```python
from build123d import *

# Parameters (mm, degrees)
SKETCH1_W           = 70
SKETCH1_H           = 60
BOSS_EXTRUDE1_DEPTH = 5.7
SKETCH2_W           = 10
SKETCH2_H           = 60
SKETCH2_R           = 2.25
BOSS_EXTRUDE2_DEPTH = 3.3
FILLET1_R           = 5
SKETCH2_4_R         = 2.5
CUT_EXTRUDE2_DEPTH  = 5


with BuildPart() as part:
    # Sketch1 → Boss-Extrude1 (new body)
    with BuildSketch(Plane(origin=(0, 0, 0), x_dir=(1, 0, 0), z_dir=(0, 1, 0))):
        Rectangle(SKETCH1_W, SKETCH1_H)
    extrude(amount=BOSS_EXTRUDE1_DEPTH)

    # Sketch2 → Boss-Extrude2 (add)
    # profile 1 of 2: a face of its own
    with BuildSketch(Plane(origin=(0, 5.7, 0), x_dir=(1, 0, 0), z_dir=(0, 1, 0))):
        with Locations((-30, 0)):
            Rectangle(SKETCH2_W, SKETCH2_H)
        with Locations(Location((-30, -25, 0), (0, 0, 270))):
            Circle(SKETCH2_R, mode=Mode.SUBTRACT)
        with Locations(Location((-30, 25, 0), (0, 0, 270))):
            Circle(SKETCH2_R, mode=Mode.SUBTRACT)
    # profile 2 of 2: a face of its own
    with BuildSketch(Plane(origin=(0, 5.7, 0), x_dir=(1, 0, 0), z_dir=(0, 1, 0))):
        with Locations((30, 0)):
            Rectangle(SKETCH2_W, SKETCH2_H)
        with Locations(Location((30, -25, 0), (0, 0, 270))):
            Circle(SKETCH2_R, mode=Mode.SUBTRACT)
        with Locations(Location((30, 25, 0), (0, 0, 90))):
            Circle(SKETCH2_R, mode=Mode.SUBTRACT)
    extrude(amount=BOSS_EXTRUDE2_DEPTH)

    # Fillet1
    fillet1_edges = [part.edges().sort_by_distance(p)[0] for p in [
        (-35, 4.5, -30),
        (-35, 4.5, 30),
        (35, 4.5, 30),
        (35, 4.5, -30),
    ]]
    fillet(fillet1_edges, radius=FILLET1_R)

    # Sketch2_4 → Cut-Extrude2 (cut)
    with BuildSketch(Plane(origin=(0, 5.7, 0), x_dir=(1, 0, 0), z_dir=(0, 1, 0))):
        with Locations(Location((-9, 5, 0), (0, 0, 270))):
            Circle(SKETCH2_4_R)
        with Locations(Location((9, 5, 0), (0, 0, 270))):
            Circle(SKETCH2_4_R)
    extrude(amount=-CUT_EXTRUDE2_DEPTH, mode=Mode.SUBTRACT)


solid = part.part
```
CAD build for the part. Positions are in the model's coordinates, mm. A direction names the side the tool comes from. Round coordinates to 2 decimals unless told otherwise and drop trailing zeros. Order: outer loops, then holes, each group sorted by start corner. A loop starts at its lowest first (then second) coordinate and runs counter-clockwise, first axis right, second up. Notation, with made-up numbers: (46.5, 8) - (62.5, 8) arc R19 cw to (62.5, 15) - close; hole circle Ø4 at (27, 15). An arc over 180 degrees is marked (long way). Answer in a Markdown table with one row per item. Add a question column.
(1) Probe L1, parallel to X at y = 1.85, z = -5; L2, parallel to X at y = 7.75, z = -1; L3, parallel to X at y = 6, z = 24.5. List the from-to ranges inside material, lowest first. Write a range as [from, to].
(2) Drop flat-ended pins along their axis: pin 1 Ø4 at (x, z) = (-8, -5) entering from +Y; pin 2 Ø7 at (x, z) = (-30, -25) entering from -Y; pin 3 Ø4 at (x, z) = (-9, -5) entering from +Y. Give the stop position or say it passes through.
(3) Mould opens along Z. For faces 1 (the face through (30, 5.7, 25)), 2 (the face through (-34, 5, 28)), 3 (the face through (-30, 9, 0)) say: +Z half, -Z half, draft (parallel to the pull), parting line (faces both ways), or undercut.
(4) 3-axis set-ups, long thin cutter, end or side, ignore diameter. For faces 4 (the face through (-31.996, 7.327, -23.962)), 5 (the face through (-35, 4, 0)), 6 (the face through (0, 5.7, 0)): which of +Z, -Z, +X, -X, +Y, -Y reach the whole face in a straight line?
(5) Band-saw the part on C-C on z = 20. List the corners of the cut face in (x, y).
(6) Band-saw the part on B-B on x = -9. List the corners of the cut face in (y, z), and give its area (3 significant figures).
(7) Band-saw the part on A-A on y = 6.5. List the corners of the cut face in (x, z).
(8) Band-saw the part on D-D on z = -5. List the corners of the cut face in (x, y).
Data:
| question | item | result |
|---|---|---|
| 1 | L1 | x = [-35, -11.5], [-6.5, 6.5], [11.5, 35] |
| 1 | L2 | x = [-35, -25], [25, 35] |
| 1 | L3 | x = [-35, -32.19], [-27.81, -25], [25, 27.81], [32.19, 35] |
| 2 | pin 1 | stops at y = 5.7 |
| 2 | pin 2 | stops at y = 0 |
| 2 | pin 3 | stops at y = 0.7 |
| 3 | face 1 | undercut |
| 3 | face 2 | +Z half |
| 3 | face 3 | draft |
| 4 | face 4 | +Y |
| 4 | face 5 | +Z, -Z, -X, +Y, -Y |
| 4 | face 6 | +Z, -Z, +Y |
| 5 | outline | (-35, 0) - (35, 0) - (35, 9) - (25, 9) - (25, 5.7) - (-25, 5.7) - (-25, 9) - (-35, 9) - close |
| 6 | outline | (0, -30) - (5.7, -30) - (5.7, -7.5) - (0.7, -7.5) - (0.7, -2.5) - (5.7, -2.5) - (5.7, 30) - (0, 30) - close |
| 6 | area | 317 mm^2 |
| 7 | outline | (-35, -25) arc R5 ccw to (-30, -30) - (-25, -30) - (-25, 30) - (-30, 30) arc R5 ccw to (-35, 25) - close; (25, -30) - (30, -30) arc R5 ccw to (35, -25) - (35, 25) arc R5 ccw to (30, 30) - (25, 30) - close; hole circle Ø4.5 at (-30, -25); hole circle Ø4.5 at (-30, 25); hole circle Ø4.5 at (30, -25); hole circle Ø4.5 at (30, 25) |
| 8 | outline | (-35, 0) - (35, 0) - (35, 9) - (25, 9) - (25, 5.7) - (11.5, 5.7) - (11.5, 0.7) - (6.5, 0.7) - (6.5, 5.7) - (-6.5, 5.7) - (-6.5, 0.7) - (-11.5, 0.7) - (-11.5, 5.7) - (-25, 5.7) - (-25, 9) - (-35, 9) - close |
